from build123d import *

# Parameters (mm, degrees)
F0_W      = 6.35
F0_H      = 6.35
F1_DEPTH  = 76.2
F3_W      = 78.9158530533
F3_H      = 6.5545327961
F4_DEPTH  = 5.08
F5_DEPTH  = 38.1
F7_DEPTH  = 25.4
F8_DEPTH  = 25.4
F9_DEPTH  = 12.7
F10_DEPTH = 12.7
F11_W     = 15.0663554668
F11_H     = 7.8755952418
F12_DEPTH = 88.9
F13_W     = 5.7417834178
F13_H     = 7.6454
F14_DEPTH = 2540
F15_W     = 5.208699964
F15_H     = 6.3248500228
F16_DEPTH = 25400


# Not quite as in the source:
# - a feature names something its author has since deleted; it is built from what else it names


with BuildPart() as f1:
    # F0 (on Top) → F1 (new body)
    with BuildSketch(Plane.XY):
        with Locations((-38.1329911691, -3.175)):
            Rectangle(F0_W, F0_H)
    extrude(amount=F1_DEPTH)

    # F3 (on face) → F4 (join)
    with BuildSketch(Plane(origin=(-6.9297761713, 0, 79.2077040846), x_dir=(0.9961946981, 0, 0.0871557427), z_dir=(0.0871557427, 0, -0.9961946981))):
        with Locations((3.0671004206, 3.2772663981)):
            Rectangle(F3_W, F3_H)
    extrude(amount=F4_DEPTH)

    # F5 (add): a face of the model
    f5_faces = [f1.faces().sort_by_distance(p)[0] for p in [
        (-42.9607486108, -3.2772663981, 73.5057000729),
    ]]
    extrude(f5_faces, amount=F5_DEPTH)

    # F6: F1 across plane


with BuildPart() as f1_1:
    add(f1.part)
    add(f1.part.mirror(Plane.YZ))

    # F7 (add): a face of the model
    f7_faces = [f1_1.faces().sort_by_distance(p)[0] for p in [
        (-41.3079911691, -3.175, 35.5502976126),
    ]]
    extrude(f7_faces, amount=F7_DEPTH)

    # F8 (add): a face of the model
    f8_faces = [f1_1.faces().sort_by_distance(p)[0] for p in [
        (41.3079911691, -3.175, 35.5502976126),
    ]]
    extrude(f8_faces, amount=F8_DEPTH)

    # F9 (add): a face of the model
    f9_faces = [f1_1.faces().sort_by_distance(p)[0] for p in [
        (0, -6.5545327961, 75.0015171841),
    ]]
    extrude(f9_faces, amount=F9_DEPTH)

    # F10 (add): faces of the model
    f10_faces = [f1_1.faces().sort_by_distance(p)[0] for p in [
        (-50.72839761, -6.35, 35.1382082279),
        (50.72839761, -6.35, 35.1382082279),
    ]]
    extrude(f10_faces, amount=F10_DEPTH)

    # F11 (on face) → F12 (cut)
    with BuildSketch(Plane(origin=(0, 0, 0), x_dir=(1, 0, 0), z_dir=(0, 0, -1))):
        with Locations((-49.9696880579, 9.0547855943)):
            Rectangle(F11_W, F11_H)
        with Locations((49.9696880579, 9.0547855943)):
            Rectangle(F11_W, F11_H)
    extrude(amount=-F12_DEPTH, mode=Mode.SUBTRACT)

    # F13 (on face) → F14 (cut)
    with BuildSketch(Plane(origin=(-66.7079911691, 0, 0), x_dir=(0, -1, 0), z_dir=(-1, 0, 0))):
        with Locations((9.922655765, 15.0297441246)):
            Rectangle(F13_W, F13_H)
    extrude(amount=-F14_DEPTH, mode=Mode.SUBTRACT)

    # F15 (on face) → F16 (cut)
    with BuildSketch(Plane(origin=(-66.7079911691, 0, 0), x_dir=(0, -1, 0), z_dir=(-1, 0, 0))):
        with Locations((9.8132924177, 58.757327497)):
            Rectangle(F15_W, F15_H)
    extrude(amount=-F16_DEPTH, mode=Mode.SUBTRACT)


solid = f1_1.part
Source: CAD feature listing. Evaluate the final solid. Frame: model axes, mm. A direction names the side the tool comes from. Give positions to 0.01 mm unless a question says otherwise; leave off trailing zeros. Write each loop counter-clockwise with the first axis right and the second up, starting at its lowest first coordinate (ties: lowest second). Pieces come first, ordered by that corner, then holes. Notation, with made-up numbers: (34, 56.25) -> (48, 56.25) arc R15 ccw to (48, 70.25) -> close; hole circle Ø11 at (85, -22). An arc over 180 degrees is marked (long way). Return JSON: item names as keys, results as strings. Group by question number.
1. Material intervals for line 1 (X direction, y = -8, z = 36); line 2 (Y direction, x = -55, z = 21); line 3 (X direction, y = -16.75, z = 7), sorted ascending. Write a range as from..to.
2. Section A-A, the plane z = 50.5. Output: boundary loops of the cut face in (x, y), then the cut area to 3 significant figures.
3. Section B-B, the plane y = -1.5. Output: boundary loops of the cut face in (x, z).
4. Mould query, pull axis Y, two halves, no side actions, for faces 1 (the face through (-66.708, -9, 34)), 2 (the face through (0, 0, 75)), 3 (the face through (51, -19.05, 35)), 4 (the face through (39, -7.052, 15)). Classes: +Y half, -Y half, draft (parallel to the pull), parting line (faces both ways), or undercut.
5. Section D-D, the plane x = -69.5. Output: boundary loops of the cut face in (y, z).
6. Section C-C, the plane x = -52. Output: boundary loops of the cut face in (y, z), then the cut area to 3 significant figures.
7. Pin query (flat end, axial travel): pin 1 Ø3.5 at (x, z) = (38.5, 13) entering from -Y; pin 2 Ø5.5 at (x, y) = (37.5, -8.5) entering from +Z; pin 3 Ø9.5 at (y, z) = (-12.5, 37.5) entering from -X; pin 4 Ø1 at (x, y) = (30.5, -3.5) entering from +Z. Return the tip coordinate at first contact, or that it passes through.
8. Access query for faces 5 (the face through (-50, -5.117, 38)), 6 (the face through (34.958, -10, 35)), 7 (the face through (62, -12.794, 15)), 8 (the face through (35.65, -9.49, 80.42)), 9 (the face through (-35.65, -9.49, 80.42)). Directions: +Z, -Z, +X, -X, +Y, -Y. A direction counts if a zero-diameter tool reaches every point of the face in a straight line with its end or side. Return the directions, or none.
Determined:
{
 "1": {"line 1": "x = -66.71..-57.5, -42.44..-34.96, 34.96..42.44, 57.5..66.71", "line 2": "y = -19.05..-12.99, -5.12..0", "line 3": "x = -66.71..-34.96, 34.96..66.71"},
 "2": {"outline": "(-66.71, -19.05) -> (-34.96, -19.05) -> (-34.96, 0) -> (-66.71, 0) -> close; (34.96, -19.05) -> (66.71, -19.05) -> (66.71, 0) -> (34.96, 0) -> close; hole (-57.5, -12.99) -> (-42.44, -12.99) -> (-42.44, -5.12) -> (-57.5, -5.12) -> close; hole (42.44, -12.99) -> (57.5, -12.99) -> (57.5, -5.12) -> (42.44, -5.12) -> close", "area": "972 mm2"},
 "3": {"outline": "(-81.14, 72.72) -> (-80.69, 67.65) -> (-66.71, 68.88) -> (-66.71, 0) -> (-34.96, 0) -> (-34.96, 71.66) -> (0, 74.71) -> (34.96, 71.66) -> (34.96, 0) -> (66.71, 0) -> (66.71, 68.88) -> (80.69, 67.65) -> (81.14, 72.72) -> (29.14, 77.26) -> (35.88, 77.85) -> (35.43, 82.91) -> (0, 79.81) -> (-35.43, 82.91) -> (-35.88, 77.85) -> (-29.14, 77.26) -> close"},
 "4": {"face 1": "draft", "face 2": "+Y half", "face 3": "-Y half", "face 4": "undercut"},
 "5": {"outline": "(-19.25, 68.63) -> (0, 68.63) -> (0, 73.73) -> (-19.25, 73.73) -> close"},
 "6": {"outline": "(-19.25, 70.17) -> (-19.05, 70.17) -> (-19.05, 0) -> (-12.99, 0) -> (-12.99, 75.26) -> (-19.25, 75.26) -> close; (-5.12, 0) -> (0, 0) -> (0, 75.26) -> (-5.12, 75.26) -> close", "area": "842 mm2"},
 "7": {"pin 1": "stops at y = -19.05", "pin 2": "stops at z = 82.91", "pin 3": "stops at x = -66.71", "pin 4": "stops at z = 82.53"},
 "8": {"face 5": "+Z, -Z", "face 6": "-Z, +Y, -Y", "face 7": "+X, -X", "face 8": "+Z, +X, +Y, -Y", "face 9": "+Z, -X, +Y, -Y"}
}
